For this review, take the finished solid that the model builds, in its own axes (mm). Face numbers are marked on the shaded views. A direction names the side the tool comes from. Round coordinates to 2 decimals unless told otherwise and drop trailing zeros. Loops run counter-clockwise (first coordinate to the right, second up) from the corner with the lowest first, then second, coordinate; pieces in that order, holes last. Notation, with made-up numbers: M 30,-7 L 51,-7 A18 cw 51,27 Z; hole C -25,-30.5 d10. An arc over 180 degrees is marked long. One line per question, with ' | ' between items. Start each with the question number.
1) Mouldability with a two-part tool opening along Y and no side actions: class the marked faces 5, 6 and 7 as pulls with the +Y half, pulls with the -Y half, needs draft (parallel to the pull), parting line crosses it, or undercut.
2) For probe 1 along Y at (x, z) = (-20, 8); probe 2 along Y at (x, z) = (-20, -6.5); probe 3 along X at (y, z) = (0, 8), list the stretches that pass through material, from the lowest coordinate up. Write a range as from..to.
3) For pin 1 Ø3 at (x, y) = (-2.5, -14.5) entering from -Z; pin 2 Ø16 at (x, y) = (4, 5.5) entering from -Z; pin 3 Ø3.5 at (y, z) = (15.5, -6) entering from +X; pin 4 Ø11 at (x, y) = (-7.5, -1.5) entering from -Z, all flat-tipped, find the tip position at first contact; note any pin that passes through.
4) We need section C-C (y = 2.5). Give the boundary of the cut face in (x, z), and give its area (3 significant figures).
5) We need section B-B (x = -5). Give the boundary of the cut face in (y, z).
6) We need section A-A (z = -5.5). Give the boundary of the cut face in (x, y), and give its area (3 significant figures).
7) For the marked faces 1, 2, 3 and 4, list the 3-axis set-ups (+Z, -Z, +X, -X, +Y, -Y) from which the entire face can be reached by the end or side of a thin tool; tool diameter is ignored.
8) We need section D-D (x = -19). Give the boundary of the cut face in (y, z).
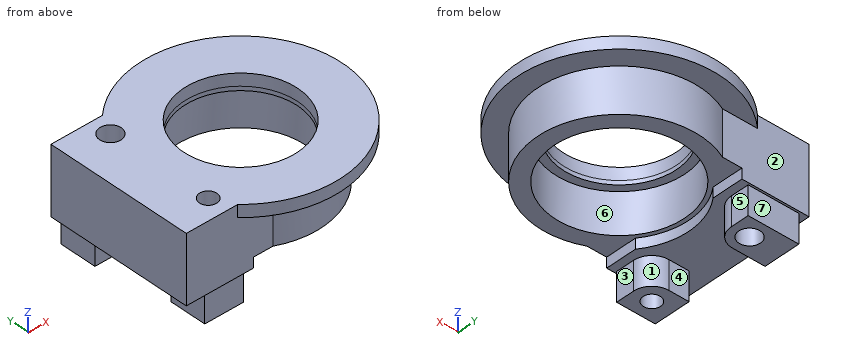
```python
from build123d import *

# Parameters (mm, degrees)
SKETCH_R        = 20
SKETCH_R_2      = 16
PAD_DEPTH       = 11
SKETCH001_R     = 25
PAD001_DEPTH    = 3
SKETCH002_R     = 16
SKETCH002_R_2   = 14
PAD002_DEPTH    = 1
SKETCH003_R     = 14
POCKET_DEPTH    = 3.001
SKETCH004_R     = 16
PAD003_DEPTH    = 14
PAD004_DEPTH    = 2.5
PAD005_DEPTH    = 7
SKETCH007_R     = 2.15
SKETCH007_R_2   = 2.65
POCKET001_DEPTH = 23.501


with BuildPart() as part:
    # Sketch → Pad (new body)
    with BuildSketch(Plane.XY):
        Circle(SKETCH_R)
        Circle(SKETCH_R_2, mode=Mode.SUBTRACT)
    extrude(amount=PAD_DEPTH)

    # Sketch001 (on Face4 of Pad) → Pad001 (join)
    with BuildSketch(Plane.XY.offset(11)):
        Circle(SKETCH001_R)
    extrude(amount=PAD001_DEPTH)

    # Sketch002 (on Face7 of Pad001) → Pad002 (join)
    with BuildSketch(Plane(origin=(0, 0, 11), x_dir=(1, 0, 0), z_dir=(0, 0, -1))):
        Circle(SKETCH002_R)
        Circle(SKETCH002_R_2, mode=Mode.SUBTRACT)
    extrude(amount=PAD002_DEPTH)

    # Sketch003 (on Face9 of Pad002) → Pocket (cut, through all)
    with BuildSketch(Plane(origin=(0, 0, 11), x_dir=(1, 0, 0), z_dir=(0, 0, -1))):
        Circle(SKETCH003_R)
    extrude(amount=-POCKET_DEPTH, mode=Mode.SUBTRACT)

    # Sketch004 (on Face6 of Pocket) → Pad003 (join)
    with BuildSketch(Plane(origin=(0, 0, 0), x_dir=(1, 0, 0), z_dir=(0, 0, -1))):
        with BuildLine():
            ThreePointArc((-8.717798, -18), (20, 0), (-8.717798, 18))
            Line((-30, 18), (-8.717798, 18))
            Line((-30, -18), (-30, 18))
            Line((-8.717798, -18), (-30, -18))
        make_face()
        Circle(SKETCH004_R, mode=Mode.SUBTRACT)
    extrude(amount=-PAD003_DEPTH)

    # Sketch005 (on Face9 of Pad003) → Pad004 (join)
    with BuildSketch(Plane(origin=(0, 0, 0), x_dir=(1, 0, 0), z_dir=(0, 0, -1))):
        with BuildLine():
            Line((-30, 18), (-13.5, 18))
            Line((-13.5, 18), (-13.5, 10.331989))
            ThreePointArc((-13.5, 10.331989), (-17, 0), (-13.5, -10.331989))
            Line((-13.5, -10.331989), (-13.5, -18))
            Line((-13.5, -18), (-30, -18))
            Line((-30, -18), (-30, 18))
        make_face()
    extrude(amount=PAD004_DEPTH)

    # Sketch006 (on Face19 of Pad004) → Pad005 (join)
    with BuildSketch(Plane(origin=(0, 0, -2.5), x_dir=(1, 0, 0), z_dir=(0, 0, -1))):
        with BuildLine():
            Line((-27.962286, -8.5), (-20.00003, -8.5))
            ThreePointArc((-15.5, -13), (-16.81803, -9.818009), (-20.00003, -8.5))
            Line((-15.5, -13), (-15.5, -17.5))
            Line((-27.962286, -17.5), (-15.5, -17.5))
            Line((-27.962286, -17.5), (-27.962286, -8.5))
        make_face()
        with BuildLine():
            Line((-25, 17.5), (-20, 17.5))
            Line((-20, 17.5), (-15.5, 17.5))
            Line((-15.5, 13), (-15.5, 17.5))
            ThreePointArc((-20, 8.5), (-16.818019, 9.818019), (-15.5, 13))
            Line((-20, 8.5), (-25, 8.5))
            Line((-25, 8.5), (-25, 17.5))
        make_face()
    extrude(amount=PAD005_DEPTH)

    # Sketch007 → Pocket001 (cut, through all)
    with BuildSketch(Plane(origin=(0, 0, -9.5), x_dir=(1, 0, 0), z_dir=(0, 0, -1))):
        with Locations((-20, 13)):
            Circle(SKETCH007_R)
        with Locations((-20, -13)):
            Circle(SKETCH007_R_2)
    extrude(amount=-POCKET001_DEPTH, mode=Mode.SUBTRACT)


solid = part.part
```
Answers below:
1) face 5: needs draft | face 6: undercut | face 7: pulls with the +Y half
2) probe 1: -18..-15.15, -10.85..10.35, 15.65..18 | probe 2: -17.5..-15.15, -10.85..-8.5, 8.5..10.35, 15.65..17.5 | probe 3: -30..-16, 16..20
3) pin 1: z = 0 | pin 2: z = 10 | pin 3: x = -15.5 | pin 4: through
4) outline: M -30,-2.5 L -16.82,-2.5 L -16.82,0 L -15.8,0 L -15.8,10 L -13.77,10 L -13.77,14 L -30,14 Z; M 13.77,10 L 15.8,10 L 15.8,0 L 19.84,0 L 19.84,11 L 24.87,11 L 24.87,14 L 13.77,14 Z | area: 320 mm^2
5) outline: M -24.49,11 L -19.36,11 L -19.36,0 L -15.2,0 L -15.2,10 L -13.08,10 L -13.08,14 L -24.49,14 Z; M 13.08,10 L 15.2,10 L 15.2,0 L 19.36,0 L 19.36,11 L 24.49,11 L 24.49,14 L 13.08,14 Z
6) outline: M -27.96,8.5 L -20,8.5 A4.5 ccw -15.5,13 L -15.5,17.5 L -27.96,17.5 Z; M -25,-17.5 L -15.5,-17.5 L -15.5,-13 A4.5 ccw -20,-8.5 L -25,-8.5 Z; hole C -20,13 d5.3; hole C -20,-13 d4.3 | area: 152 mm^2
7) face 1: -Z, +X | face 2: -Z, -X, +Y | face 3: -Z, +X, +Y, -Y | face 4: -Z, +X, -X
8) outline: M -18,-2.5 L -17.5,-2.5 L -17.5,-9.5 L -14.9,-9.5 L -14.9,14 L -18,14 Z; M -11.1,-9.5 L -8.61,-9.5 L -8.61,-2.5 L 8.61,-2.5 L 8.61,-9.5 L 10.55,-9.5 L 10.55,14 L -11.1,14 Z; M 15.45,-9.5 L 17.5,-9.5 L 17.5,-2.5 L 18,-2.5 L 18,14 L 15.45,14 Z
